Answer from the drawing. Dimensions are ordinates in mm from the lowest x, y and z of the part. Coordinates: 2 decimals unless noted, no trailing zeros. Write each loop counter-clockwise with the first axis right and the second up, starting at its lowest first coordinate (ties: lowest second). Pieces come first, ordered by that corner, then holes. Notation, with made-up numbers: (13, 46) - (51, 46) arc R10 cw to (51, 62) - close; hole circle Ø4 at (63.25, 70). An arc over 180 degrees is marked (long way). Use a Markdown table: item, result.
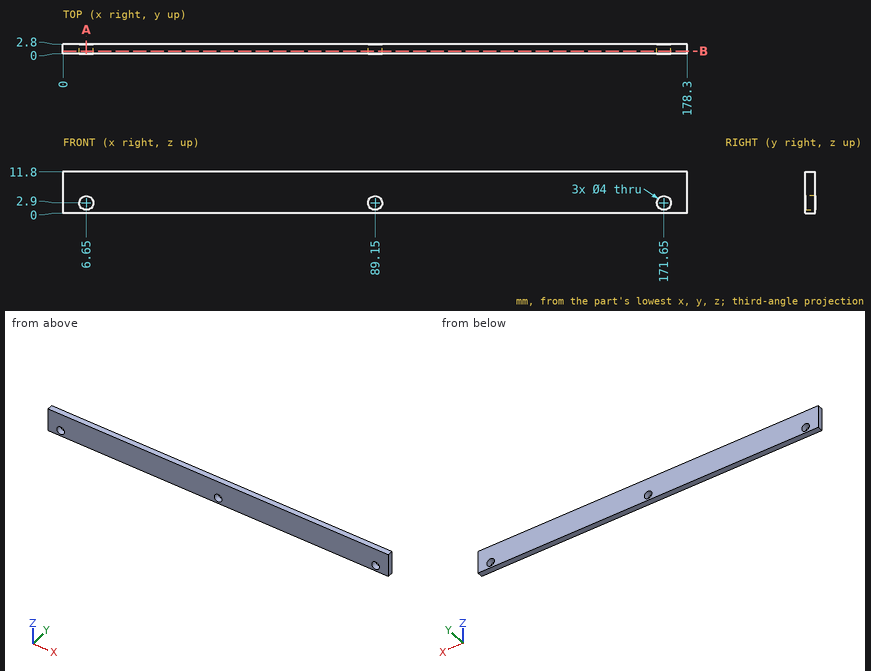
(1) A cutting plane is placed at A-A, the plane x = 6.65. Write down the section's boundary in (y, z), and give its area (3 significant figures).
Report:
| item | result |
|---|---|
| outline | (0, 0) - (2.8, 0) - (2.8, 0.9) - (0, 0.9) - close; (0, 4.9) - (2.8, 4.9) - (2.8, 11.8) - (0, 11.8) - close |
| area | 21.8 mm² |
(2) Straight lines are drawn through the part: L1, parallel to X at y = 0.8, z = 2.9; L2, parallel to Z at x = 89.15, y = 1.7; L3, parallel to X at y = 0.65, z = 4. For each, find the intervals that lie inside material, in ascending order.
Report:
| item | result |
|---|---|
| L1 | x = 0 to 4.65, 8.65 to 87.15, 91.15 to 169.65, 173.65 to 178.3 |
| L2 | z = 0 to 0.9, 4.9 to 11.8 |
| L3 | x = 0 to 4.98, 8.32 to 87.48, 90.82 to 169.98, 173.32 to 178.3 |
(3) A cutting plane is placed at B-B, the plane y = 0.75. Write down the section's boundary in (x, z).
Report:
| item | result |
|---|---|
| outline | (0, 0) - (178.3, 0) - (178.3, 11.8) - (0, 11.8) - close; hole circle Ø4 at (6.65, 2.9); hole circle Ø4 at (89.15, 2.9); hole circle Ø4 at (171.65, 2.9) |
